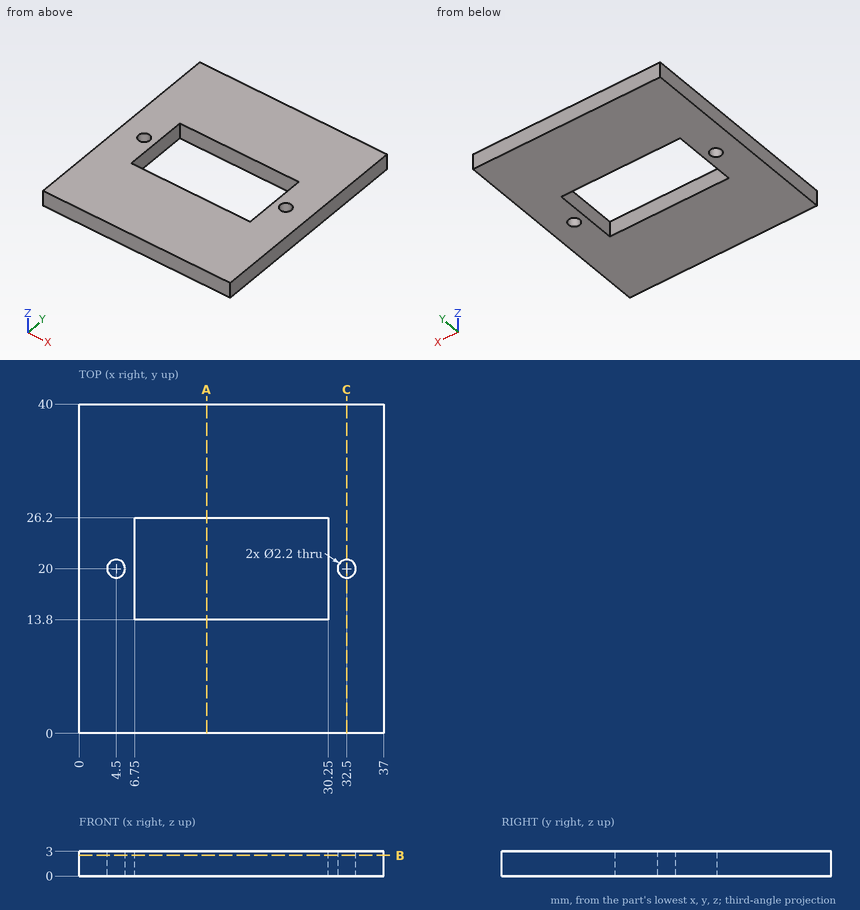
For this review, use the dimensioned drawing (mm, ordinates from the lowest corner) and the shaded views. Coordinates: 2 decimals unless noted, no trailing zeros. Loops run counter-clockwise (first coordinate to the right, second up) from the corner with the lowest first, then second, coordinate; pieces in that order, holes last. Notation, with made-up numbers: (-32.75, 41.25) -> (-18.75, 41.25) arc R8 cw to (-18.75, 46.25) -> close; hole circle Ø5 at (5.5, 39). An arc over 180 degrees is marked (long way). Use a Markdown table: item, result. Add a question column.
Item 1: We need section B-B, the plane z = 2.5. Write out the cut boundary in (x, y).
Item 2: We need section A-A, the plane x = 15.5. Write out the cut boundary in (y, z), and give its area (3 significant figures).
Item 3: Wall thickness on L1, parallel to Y at x = 27, z = 2.85; L2, parallel to Y at x = 32.5, z = 1.8; L3, parallel to X at y = 24, z = 1.7: over which ranges is each line inside the solid? List them lowest first. Write a range as from..to.
Item 4: We need section C-C, the plane x = 32.5. Write out the cut boundary in (y, z).
Numbers:
| question | item | result |
|---|---|---|
| 1 | outline | (0, 0) -> (37, 0) -> (37, 40) -> (0, 40) -> close; hole circle Ø2.2 at (4.5, 20); hole (6.75, 13.8) -> (30.25, 13.8) -> (30.25, 26.2) -> (6.75, 26.2) -> close; hole circle Ø2.2 at (32.5, 20) |
| 2 | outline | (0, 0) -> (13.8, 0) -> (13.8, 3) -> (0, 3) -> close; (26.2, 0) -> (40, 0) -> (40, 3) -> (26.2, 3) -> close |
| 2 | area | 82.8 mm^2 |
| 3 | L1 | y = 0..13.8, 26.2..40 |
| 3 | L2 | y = 0..18.9, 21.1..40 |
| 3 | L3 | x = 0..6.75, 30.25..37 |
| 4 | outline | (0, 0) -> (18.9, 0) -> (18.9, 3) -> (0, 3) -> close; (21.1, 0) -> (40, 0) -> (40, 3) -> (21.1, 3) -> close |
